from build123d import *

# Parameters (mm, degrees)
SKETCH1_R           = 5
BOSS_EXTRUDE1_DEPTH = 60.5
SKETCH24_R          = 5
SKETCH24_R_2        = 4.5
CUT_EXTRUDE3_DEPTH  = 2.5
SKETCH25_R          = 5
SKETCH25_R_2        = 4.5
CUT_EXTRUDE4_DEPTH  = 2.5


with BuildPart() as part:
    # Sketch1 → Boss-Extrude1 (new body)
    with BuildSketch(Plane(origin=(0, 0, 0), x_dir=(1, 0, 0), z_dir=(0, 1, 0))):
        Circle(SKETCH1_R)
    extrude(amount=BOSS_EXTRUDE1_DEPTH)

    # Sketch24 → Cut-Extrude3 (cut)
    with BuildSketch(Plane(origin=(0, 0, 0), x_dir=(-1, 0, 0), z_dir=(0, -1, 0))):
        Circle(SKETCH24_R)
        Circle(SKETCH24_R_2, mode=Mode.SUBTRACT)
    extrude(amount=-CUT_EXTRUDE3_DEPTH, mode=Mode.SUBTRACT)

    # Sketch25 → Cut-Extrude4 (cut)
    with BuildSketch(Plane(origin=(0, 60.5, 0), x_dir=(1, 0, 0), z_dir=(0, 1, 0))):
        Circle(SKETCH25_R)
        Circle(SKETCH25_R_2, mode=Mode.SUBTRACT)
    extrude(amount=-CUT_EXTRUDE4_DEPTH, mode=Mode.SUBTRACT)


solid = part.part
Source: CAD feature listing. Evaluate the final solid. Frame: model axes, mm. A direction names the side the tool comes from. Give positions to 0.01 mm unless a question says otherwise; leave off trailing zeros. Write each loop counter-clockwise with the first axis right and the second up, starting at its lowest first coordinate (ties: lowest second). Pieces come first, ordered by that corner, then holes. Notation, with made-up numbers: M -28.75,13.5 L 11.25,13.5 A20 ccw 11.25,17.5 Z; hole C 30.25,36 d8. An arc over 180 degrees is marked long. Return JSON: item names as keys, results as strings. Group by question number.
1) Set-up query: faces 1 (the face through (0.59, 1.23, -4.46)), 2 (the face through (-1.08, 29.86, 4.88)), 3 (the face through (-0.59, 59.27, -4.46)). Return all of +Z, -Z, +X, -X, +Y, -Y with unobstructed straight access to the full face (end or side cutting, diameter ignored); none if empty.
2) Cut plane A-A, the plane z = 4. Output: boundary loops of the cut face in (x, y), then the cut area to 3 significant figures.
3) Ray query, L1, parallel to Y at x = -2.5, z = 4.25; L2, parallel to X at y = 17.5, z = -0.25; L3, parallel to Z at x = 2, y = 44.5. Return the intervals inside material, ascending.
4) First-contact query: pin 1 Ø5 at (x, z) = (-1.5, 1.5) entering from -Y; pin 2 Ø3 at (x, y) = (-2, 28.5) entering from +Z. Flat tips, straight axial feed; report the tip coordinate or a pass-through.
5) Cut plane B-B, the plane x = -2. Output: boundary loops of the cut face in (y, z), then the cut area to 3 significant figures.
6) Cut plane C-C, the plane y = 7.5. Output: boundary loops of the cut face in (x, z).
Data:
{
 "1": {"face 1": "-Y", "face 2": "+Y, -Y", "face 3": "+Y"},
 "2": {"outline": "M -3,2.5 L -2.06,2.5 L -2.06,0 L 2.06,0 L 2.06,2.5 L 3,2.5 L 3,58 L 2.06,58 L 2.06,60.5 L -2.06,60.5 L -2.06,58 L -3,58 Z", "area": "354 mm²"},
 "3": {"L1": "y = 2.5 to 58", "L2": "x = -4.99 to 4.99", "L3": "z = -4.58 to 4.58"},
 "4": {"pin 1": "stops at y = 0", "pin 2": "stops at z = 4.97"},
 "5": {"outline": "M 0,-4.03 L 2.5,-4.03 L 2.5,-4.58 L 58,-4.58 L 58,-4.03 L 60.5,-4.03 L 60.5,4.03 L 58,4.03 L 58,4.58 L 2.5,4.58 L 2.5,4.03 L 0,4.03 Z", "area": "549 mm²"},
 "6": {"outline": "C 0,0 d10"}
}
